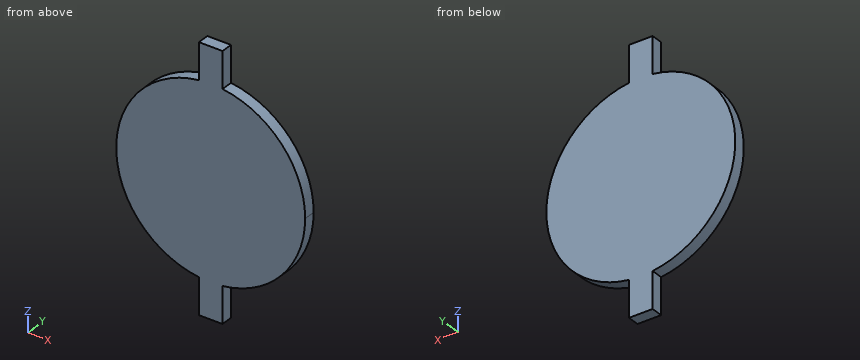
from build123d import *

# Parameters (mm, degrees)
BOSS_EXTRUDE1_DEPTH = 5


with BuildPart() as part:
    # Sketch1 → Boss-Extrude1 (new body)
    with BuildSketch(Plane(origin=(0, 0, 0), x_dir=(1, 0, 0), z_dir=(0, 1, 0))):
        with BuildLine():
            ThreePointArc((-5, 39.686269666), (-40, 0), (-5, -39.686269666))
            Line((-5, -39.686269666), (-5, 39.686269666))
        make_face()
        with BuildLine():
            ThreePointArc((-5, 39.686269666), (0, 40), (5, 39.686269666))
            Line((5, 39.686269666), (5, 55))
            Line((5, 55), (-5, 55))
            Line((-5, 55), (-5, 39.686269666))
        make_face()
        with BuildLine():
            Line((5, 39.686269666), (5, -39.686269666))
            ThreePointArc((5, -39.686269666), (30, -26.457513111), (40, 0))
            ThreePointArc((40, 0), (30, 26.457513111), (5, 39.686269666))
        make_face()
        with BuildLine():
            ThreePointArc((-5, -39.686269666), (0, -40), (5, -39.686269666))
            Line((5, -39.686269666), (5, 39.686269666))
            ThreePointArc((5, 39.686269666), (0, 40), (-5, 39.686269666))
            Line((-5, 39.686269666), (-5, -39.686269666))
        make_face()
        with BuildLine():
            Line((-5, -55), (5, -55))
            Line((5, -55), (5, -39.686269666))
            ThreePointArc((5, -39.686269666), (0, -40), (-5, -39.686269666))
            Line((-5, -39.686269666), (-5, -55))
        make_face()
    extrude(amount=BOSS_EXTRUDE1_DEPTH)


solid = part.part
The listing builds one solid part. Answer for the finished solid, in the listing's coordinates (mm). Coordinates: 2 decimals unless noted, no trailing zeros. Write each loop counter-clockwise with the first axis right and the second up, starting at its lowest first coordinate (ties: lowest second). Pieces come first, ordered by that corner, then holes. Notation, with made-up numbers: M -10.5,-5.75 L 34.5,-5.75 A9 cw 34.5,8.25 Z; hole C -23,-25 d9. An arc over 180 degrees is marked long. Put each result on its own line as item: value. Start each with the question number.
1. A cutting plane is placed at A-A on y = 1.2. Write down the section's boundary in (x, z), then the cut area to 3 significant figures.
2. Flat-ended cylindrical pins translate along their axes: P1, Ø8, axis at x = -15, z = 32.5, coming from the -Y side; P2, Ø1.5, axis at y = 4, z = 1, coming from the -X side; P3, Ø1.5, axis at y = 1.5, z = -49.5, coming from the -X side; P4, Ø1.5, axis at y = 3.5, z = 28, coming from the -X side. Find the tip coordinate at first contact, or state that the pin passes through.
3. Consider line 1 (X direction, y = 3.7, z = 50); line 2 (Z direction, x = -13.5, y = 1.1); line 3 (Z direction, x = -17, y = 4.1). Determine where each line is inside the solid, lowest interval first. Write a range as from..to.
4. A cutting plane is placed at C-C on x = 24.5. Write down the section's boundary in (y, z), then the cut area to 3 significant figures.
5. A cutting plane is placed at B-B on z = 35.5. Write down the section's boundary in (x, y), then the cut area to 3 significant figures.
Resolved:
1. outline: M -5,-55 L 5,-55 L 5,-39.69 A40 ccw 5,39.69 L 5,55 L -5,55 L -5,39.69 A40 ccw -5,-39.69 Z
1. area: 5,330 mm2
2. P1: stops at y = 0
2. P2: stops at x = -40
2. P3: stops at x = -5
2. P4: stops at x = -29.28
3. line 1: x = -5..5
3. line 2: z = -37.65..37.65
3. line 3: z = -36.21..36.21
4. outline: M 0,-31.62 L 5,-31.62 L 5,31.62 L 0,31.62 Z
4. area: 316 mm2
5. outline: M -18.43,0 L 18.43,0 L 18.43,5 L -18.43,5 Z
5. area: 184 mm2
